Input: part model. Units: mm. Frame: model coordinates. Face numbers are marked on the shaded views. A direction names the side the tool comes from. Coordinates: 2 decimals unless noted, no trailing zeros. Loops run counter-clockwise (first coordinate to the right, second up) from the corner with the lowest first, then second, coordinate; pieces in that order, holes last. Notation, with made-up numbers: (8.5, -40) - (27.5, -40) arc R24 ccw to (27.5, -17) - close; hole circle Ø8 at (-6, -34.75). An arc over 180 degrees is marked (long way). Use a Markdown table: item, result. Add a question column.
1. Ray query, L1, parallel to Y at x = -8, z = 2; L2, parallel to Z at x = 21, y = -1.5. Return the intervals inside material, ascending. Write a range as [from, to].
2. Section query C-C on z = -13.5. Return the cut outline in (x, y).
3. Section query B-B on x = -13.5. Return the cut outline in (y, z), then the cut area to 3 significant figures.
4. Access query for the marked faces 1, 2, 3, 4 and 5. Directions: +Z, -Z, +X, -X, +Y, -Y. A direction counts if a zero-diameter tool reaches every point of the face in a straight line with its end or side. Return the directions, or none.
5. Section query A-A on y = -3.5. Return the cut outline in (x, z).
6. Section query D-D on x = 0. Return the cut outline in (y, z), then the cut area to 3 significant figures.
7. Contact query for flat-ended pins moving along their axis: P1, Ø8, axis at x = -9.5, y = -9.5, coming from the +Z side; P2, Ø1, axis at x = -15.5, z = 9, coming from the -Y side; P3, Ø4, axis at x = -21, y = -9.5, coming from the +Z side. Output: stop coordinate, or through.
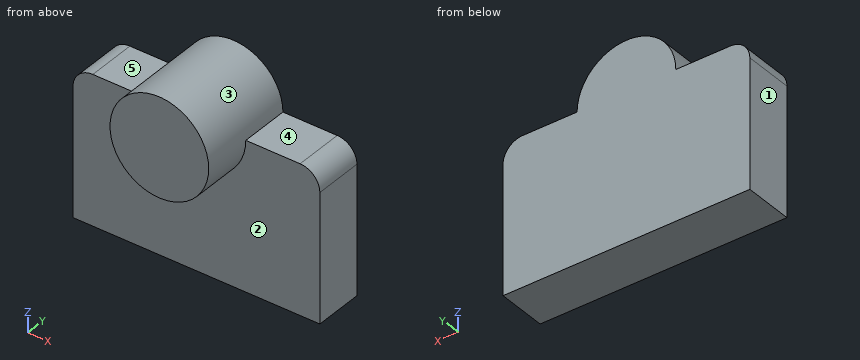
```python
from build123d import *

# Parameters (mm, degrees)
F0_W     = 63.5
F0_H     = 38.1
F1_DEPTH = 12.7
F2_R     = 5.08
F3_R     = 12.7
F4_DEPTH = 25.4


with BuildPart() as f1:
    # F0 (on Front) → F1 (new body)
    with BuildSketch(Plane.XZ):
        Rectangle(F0_W, F0_H)
    extrude(amount=F1_DEPTH)

    # F2
    f2_edges = [f1.edges().sort_by_distance(p)[0] for p in [
        (31.75, -6.35, 19.05),
        (-31.75, -6.35, 19.05),
    ]]
    fillet(f2_edges, radius=F2_R)

    # F3 (on Front) → F4 (join)
    with BuildSketch(Plane.XZ):
        with Locations((0, 19.05)):
            Circle(F3_R)
    extrude(amount=F4_DEPTH)


solid = f1.part
```
Resolved:
| question | item | result |
|---|---|---|
| 1 | L1 | [-12.7, 0] |
| 1 | L2 | [-19.05, 19.05] |
| 2 | outline | (-31.75, -12.7) - (31.75, -12.7) - (31.75, 0) - (-31.75, 0) - close |
| 3 | outline | (-12.7, -19.05) - (0, -19.05) - (0, 19.05) - (-12.7, 19.05) - close |
| 3 | area | 484 mm² |
| 4 | face 1 | +Z, -Z, -X, +Y, -Y |
| 4 | face 2 | -Z, -Y |
| 4 | face 3 | -Y |
| 4 | face 4 | +Z, +X, +Y, -Y |
| 4 | face 5 | +Z, -X, +Y, -Y |
| 5 | outline | (-31.75, -19.05) - (31.75, -19.05) - (31.75, 13.97) arc R5.08 ccw to (26.67, 19.05) - (12.7, 19.05) arc R12.7 ccw to (-12.7, 19.05) - (-26.67, 19.05) arc R5.08 ccw to (-31.75, 13.97) - close |
| 6 | outline | (-25.4, 6.35) - (-12.7, 6.35) - (-12.7, -19.05) - (0, -19.05) - (0, 31.75) - (-25.4, 31.75) - close |
| 6 | area | 968 mm² |
| 7 | P1 | z = 30.5 |
| 7 | P2 | y = -12.7 |
| 7 | P3 | z = 19.05 |
